The figure shows three views and two pictorial views of one solid part (mm, origin at its lowest corner). Answer the questions. A direction names the side the tool comes from. Give positions to 0.01 mm unless a question says otherwise; leave off trailing zeros. Write each loop counter-clockwise with the first axis right and the second up, starting at its lowest first coordinate (ties: lowest second). Pieces come first, ordered by that corner, then holes. Notation, with made-up numbers: M 40,7 L 44,7 A33 cw 44,38 Z; hole C -9.5,33 d8. An arc over 180 degrees is marked long. Return JSON: item names as keys, results as strings.
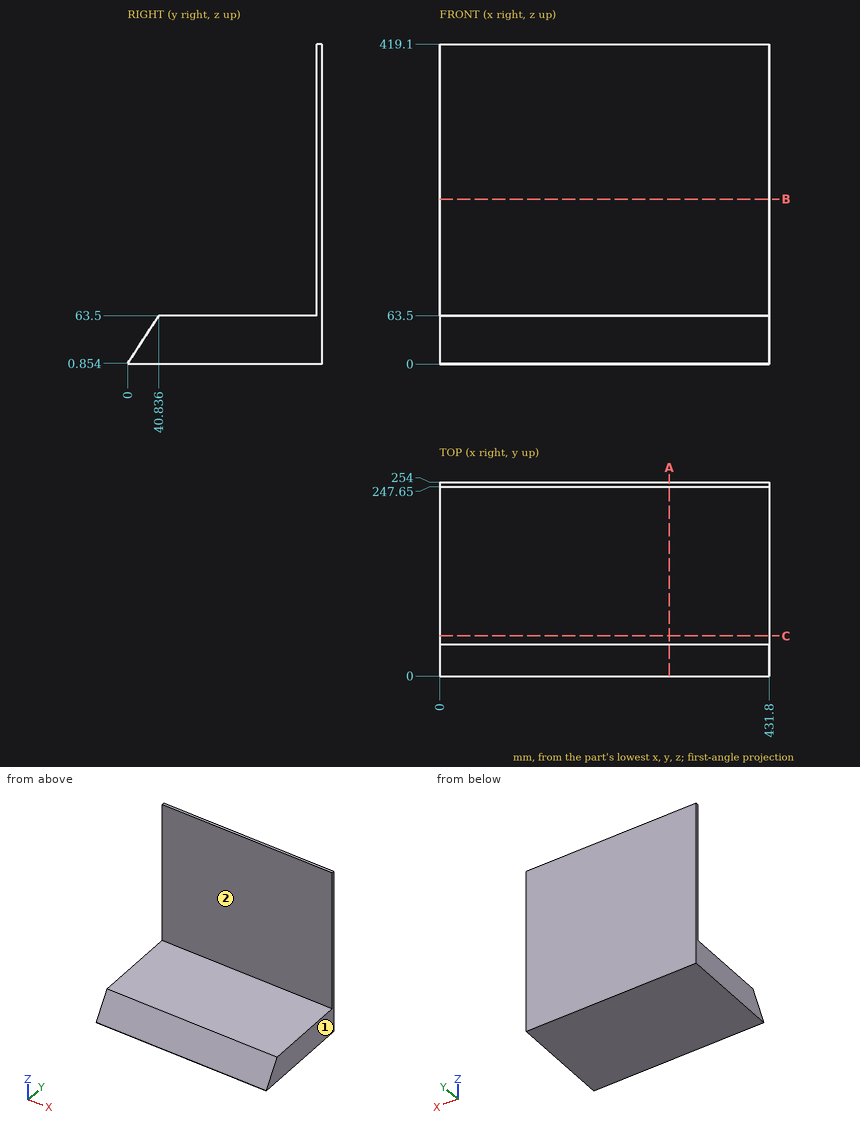
Item 1: A cutting plane is placed at A-A, the plane x = 301. Write down the section's boundary in (y, z), plus the area to 3 significant figures.
Geometry results:
{"outline": "M 0,0 L 254,0 L 254,419.1 L 247.65,419.1 L 247.65,63.5 L 40.84,63.5 L 0,0.85 Z", "area": "17,100 mm2"}
Item 2: Find the intervals of material crossed by line 1 (Z direction, x = 411, y = 114.5); line 2 (Y direction, x = 128, z = 68); line 3 (Y direction, x = 342, z = 17.5), in increasing order.
Geometry results:
{"line 1": "z = 0 to 63.5", "line 2": "y = 247.65 to 254", "line 3": "y = 10.85 to 254"}
Item 3: Which of the six approach directions +Z, -Z, +X, -X, +Y, -Y give full straight-line access (tool end or side, diameter ignored) to the marked faces 1 and 2?
Geometry results:
{"face 1": "+Z, -Z, +X, +Y, -Y", "face 2": "+Z, +X, -X, -Y"}
Item 4: A cutting plane is placed at C-C, the plane y = 52.5. Write down the section's boundary in (x, z).
Geometry results:
{"outline": "M 0,0 L 431.8,0 L 431.8,63.5 L 0,63.5 Z"}
Item 5: A cutting plane is placed at B-B, the plane z = 216. Write down the section's boundary in (x, y).
Geometry results:
{"outline": "M 0,247.65 L 431.8,247.65 L 431.8,254 L 0,254 Z"}
Item 6: Given pin 1 Ø4 at (x, z) = (164, 95.5) entering from -Y; pin 2 Ø3 at (x, z) = (358.5, 53.5) entering from -Y, each flat-ended and moving along its own axis, determine where each tip first touches the part or whether it passes through.
Geometry results:
{"pin 1": "stops at y = 247.65", "pin 2": "stops at y = 33.34"}
